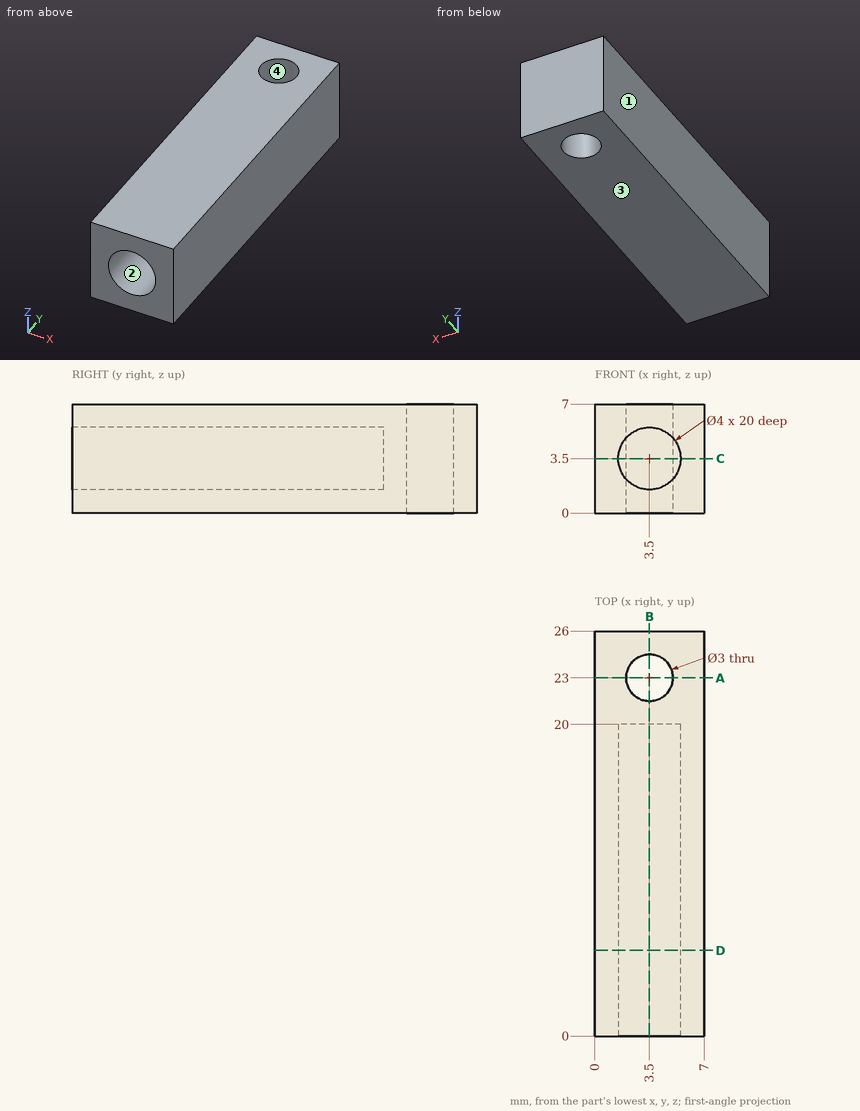
Could you check a few things on this drawing? It's one solid part, dimensions in mm from its lowest x, y, z. Coordinates: 2 decimals unless noted, no trailing zeros. Loops run counter-clockwise (first coordinate to the right, second up) from the corner with the lowest first, then second, coordinate; pieces in that order, holes last.
1. Imagine slicing it at A-A (y = 23). Please give me the cut outline in (x, z), and give its area (3 significant figures).
2. We'd pull the mould along X, two halves only. Please class the marked faces 1, 2, 3 and 4: released by +X, released by -X, zero draft, split by the parting line, or undercut.
3. Imagine slicing it at C-C (z = 3.5). Please give me the cut outline in (x, y), and give its area (3 significant figures).
4. Imagine slicing it at D-D (y = 5.5). Please give me the cut outline in (x, z).
5. I need wall thicknesses on L1, parallel to Y at x = 3.5, z = 4; L2, parallel to Z at x = 3.5, y = 7.25. Which ranges of each line are inside material? Lowest first, please.
6. Imagine slicing it at B-B (x = 3.5). Please give me the cut outline in (y, z).
Computed values:
1. outline: (0, 0) - (2, 0) - (2, 7) - (0, 7) - close; (5, 0) - (7, 0) - (7, 7) - (5, 7) - close
1. area: 28.0 mm2
2. face 1: released by -X
2. face 2: undercut
2. face 3: zero draft
2. face 4: undercut
3. outline: (0, 0) - (1.5, 0) - (1.5, 20) - (5.5, 20) - (5.5, 0) - (7, 0) - (7, 26) - (0, 26) - close; hole circle Ø3 at (3.5, 23)
3. area: 94.9 mm2
4. outline: (0, 0) - (7, 0) - (7, 7) - (0, 7) - close; hole circle Ø4 at (3.5, 3.5)
5. L1: y = 20 to 21.5, 24.5 to 26
5. L2: z = 0 to 1.5, 5.5 to 7
6. outline: (0, 0) - (21.5, 0) - (21.5, 7) - (0, 7) - (0, 5.5) - (20, 5.5) - (20, 1.5) - (0, 1.5) - close; (24.5, 0) - (26, 0) - (26, 7) - (24.5, 7) - close
